Autodesk Fusion 360 part; units mm, degrees
sketch "Sketch1" plane through (0, 0, 0) normal (0, 1, 0) x (1, 0, 0)
  circle A0 centre (0, 0) radius 1.9
  circle A1 centre (0, 0) radius 4
  dimension "d1" = 3.8
  dimension "d2" = 8
extrude "Extrude1" add sketch "Sketch1" along normal blind 22
chamfer "Chamfer2" distance 0.5 angle 45 1 edges at (-1.7714, 0, -0.6871)
sketch "Sketch2" plane through (0, 22, 0) normal (0, 1, 0) x (-1, 0, 0)
  circle A0 centre (0, 0) radius 1.9
  circle A1 centre (0, 0) radius 4
  circle A2 centre (0, 0) radius 6
  line L0 (3.5, 2.0207) -> (0, 4.0415)
  line L1 (0, 4.0415) -> (-3.5, 2.0207)
  line L2 (-3.5, 2.0207) -> (-3.5, -2.0207)
  line L3 (-3.5, -2.0207) -> (0, -4.0415)
  line L4 (0, -4.0415) -> (3.5, -2.0207)
  line L5 (3.5, -2.0207) -> (3.5, 2.0207)
  circle A3 centre (0, 0) radius 2.25
  dimension "d7" = 12
  dimension "d8" = 3.5
  dimension "d9" = 4.5
extrude "Extrude3" cut sketch "Sketch2" against normal blind 3 contours A1 L0 L1 L2 L3 L4 L5 | A3
extrude "Extrude2" add sketch "Sketch2" against normal blind 8 contours A1 L0 L5 | A1 L4 L5 | A1 L0 L1 | A1 L3 L4 | A1 L1 L2 | A1 L2 L3 | A2
extrude "Extrude4" cut sketch "Sketch2" against normal blind 10 contours A3
chamfer "Chamfer3" distance 2 angle 45 1 edges at (5.594, 14, 2.1697)
chamfer "Chamfer4" distance 0.3 angle 45 1 edges at (-1.7714, 12, 0.6871)
Here's how the part is built. I have some questions about the finished solid (model axes, mm). A direction names the side the tool comes from. Give positions to 0.01 mm unless a question says otherwise; leave off trailing zeros. Write each loop counter-clockwise with the first axis right and the second up, starting at its lowest first coordinate (ties: lowest second). Pieces come first, ordered by that corner, then holes. Notation, with made-up numbers: (49.25, 46) -> (80.25, 46) arc R34 cw to (80.25, 79) -> close; hole circle Ø11 at (19, -6). An arc over 180 degrees is marked (long way). Write each question's results on one line, items separated by ' | '.
Item 1: If I drill on L1, parallel to Z at x = 0, y = 3; L2, parallel to Z at x = 0, y = 17.25, over which ranges is the centre line in solid material (lowest first)?
Output:
L1: z = -4 to -1.9, 1.9 to 4 | L2: z = -6 to -2.25, 2.25 to 6
Item 2: On a 3-axis mill with a long thin cutter (end or side, diameter ignored), from which of +Z, -Z, +X, -X, +Y, -Y can I reach the whole of each face in a straight line? I mean faces 1 (the face through (-0.867, 6.902, -3.905)), 2 (the face through (2, 0, 2)), 3 (the face through (0.29, 15.55, 2.23)). Say none if no direction works.
Output:
face 1: -Y | face 2: +Z, -Z, +X, -X, -Y | face 3: +Y
Item 3: Suppose I cut it at B-B on y = 16.5. Write out the boundary of the cut face in (x, z).
Output:
outline: circle Ø12 at (0, 0); hole circle Ø4.5 at (0, 0)
Item 4: For pin 1 Ø3 at (y, z) = (4, 1) entering from +X; pin 2 Ø2 at (x, y) = (4, 17.5) entering from -Z; pin 3 Ø2 at (x, z) = (0, 1) entering from +Y, each with a flat end and sliding along its axis, tell me the tip position at first contact or that it passes through.
Output:
pin 1: stops at x = 4 | pin 2: stops at z = -5.2 | pin 3: stops at y = 11.8
Item 5: Suppose I cut it at C-C on y = 3.25. Write out the boundary of the cut face in (x, z).
Output:
outline: circle Ø8 at (0, 0); hole circle Ø3.8 at (0, 0)
